```python
from build123d import *

# Parameters (mm, degrees)
PAD001_DEPTH      = 11
FILLET001_R       = 1.2
SKETCH005_W       = 6.70052
SKETCH005_H       = 40.2844
SKETCH006_R       = 5.25
POCKET_DEPTH      = 0.001
POCKET_DEPTH_BACK = 143.4094


with BuildPart() as part:
    # Sketch004 → Pad001 (new body)
    with BuildSketch(Plane.XZ.offset(-6.7)):
        with BuildLine():
            Line((-6.70052, 141.8844), (-9.6647, 143.4084))
            ThreePointArc((-9.6647, 143.4084), (-17.256712, 140.927389), (-24.479189, 137.517128))
            ThreePointArc((-24.479189, 137.517128), (-25.118047, 135.6415), (-23.310129, 134.830602))
            ThreePointArc((-6.70052, 127), (-13.446839, 134.221029), (-23.310129, 134.830602))
            Line((0, 127), (-6.70052, 127))
            Line((0, 141.8844), (0, 127))
            Line((-6.70052, 141.8844), (0, 141.8844))
        make_face()
    pad001 = extrude(amount=PAD001_DEPTH)

    # Mirrored: Pad001 across Sketch004 V_Axis
    add(pad001.mirror(Plane(origin=(0, 6.7, 0), x_dir=(0, -1, 0), z_dir=(1, 0, 0))))

    # Fillet001
    fillet001_edges = [part.edges().sort_by_distance(p)[0] for p in [
        (17.256712, 6.7, 140.927389),
        (17.256712, -4.3, 140.927389),
        (-17.256712, -4.3, 140.927389),
        (-17.256712, 6.7, 140.927389),
    ]]
    fillet(fillet001_edges, radius=FILLET001_R)

    # Sketch005 → Revolution (revolve)
    with BuildSketch(Plane.XZ):
        with Locations((-3.35026, 121.7422)):
            Rectangle(SKETCH005_W, SKETCH005_H)
    revolve(axis=Axis((0, 0, 0), (0, 0, 1)))

    # Sketch006 → Pocket (cut, two sides)
    with BuildSketch(Plane.XY) as pocket_sk:
        Circle(SKETCH006_R)
    extrude(amount=-POCKET_DEPTH, mode=Mode.SUBTRACT)
    extrude(pocket_sk.sketch, amount=POCKET_DEPTH_BACK, mode=Mode.SUBTRACT)


solid = part.part
```
Here's how the part is built. I have some questions about the finished solid (model axes, mm). A direction names the side the tool comes from. Coordinates: 2 decimals unless noted, no trailing zeros. Loops run counter-clockwise (first coordinate to the right, second up) from the corner with the lowest first, then second, coordinate; pieces in that order, holes last. Notation, with made-up numbers: M -39.75,11.25 L -22.75,11.25 A29 ccw -22.75,38.25 Z; hole C -4,45 d8. An arc over 180 degrees is marked long. One line per item, written item: value.
1. Thinking about a two-plate mould opening in X: for faces 1 (the flat face through (7, 6.7, 137)), 2 (the flat face through (-8.162, 1.277, 142.636)), 3 (the cylindrical face through (0.872, -6.644, 117.548)), which applies, +X half, -X half, draft (parallel to the pull), parting line (faces both ways), or undercut?
Geometry says:
face 1: draft
face 2: undercut
face 3: parting line
2. Will these pins go through, and if not, where does the flat tip stop? pin 1 Ø2 at (x, y) = (2, 4) entering from -Z; pin 2 Ø5 at (y, z) = (-1, 107) entering from +X; pin 3 Ø6.5 at (x, y) = (0.5, 2.5) entering from +Z; pin 4 Ø8 at (x, z) = (-14.5, 137.5) entering from -Y.
Geometry says:
pin 1: stops at z = 101.6
pin 2: stops at x = 6.7
pin 3: stops at z = 141.88
pin 4: stops at y = -4.3
3. Imagine slicing it at C-C (y = 4.25). List the corners of the cut face in (x, z) for me.
Geometry says:
outline: M -24.48,137.52 A1.47 ccw -23.31,134.83 A13.36 cw -6.7,127 L -5.18,127 L -5.18,101.6 L -3.08,101.6 L -3.08,141.88 L -6.7,141.88 L -9.66,143.41 A63.79 ccw Z; M 3.08,101.6 L 5.18,101.6 L 5.18,127 L 6.7,127 A13.36 cw 23.31,134.83 A1.47 ccw 24.48,137.52 A63.79 ccw 9.66,143.41 L 6.7,141.88 L 3.08,141.88 Z
4. Imagine slicing it at B-B (z = 125). List the corners of the cut face in (x, y) for me.
Geometry says:
outline: C 0,0 d13.4; hole C 0,0 d10.5
5. On a 3-axis mill with a long thin cutter (end or side, diameter ignored), from which of +Z, -Z, +X, -X, +Y, -Y can I reach the whole of each face in a straight line? I mean faces 4 (the flat face through (-5, 5, 127)), 5 (the flat face through (8.162, 1.277, 142.636)), 6 (the flat face through (-6.2, -3.1, 127)). Say none if no direction works.
Geometry says:
face 4: -Z, -X, +Y
face 5: +Z, +Y, -Y
face 6: -Z, -X, -Y
6. Please list where these lines run through material, in increasing order: probe 1 along X at (y, z) = (0, 113.5); probe 2 along Y at (x, z) = (18, 138).
Geometry says:
probe 1: x = -6.7 to -5.25, 5.25 to 6.7
probe 2: y = -4.3 to 6.7
7. Imagine slicing it at A-A (y = 1). List the corners of the cut face in (x, z) for me.
Geometry says:
outline: M -24.48,137.52 A1.47 ccw -23.31,134.83 A13.36 cw -6.7,127 L -6.63,127 L -6.63,101.6 L -5.15,101.6 L -5.15,141.88 L -6.7,141.88 L -9.66,143.41 A63.79 ccw Z; M 5.15,101.6 L 6.63,101.6 L 6.63,127 L 6.7,127 A13.36 cw 23.31,134.83 A1.47 ccw 24.48,137.52 A63.79 ccw 9.66,143.41 L 6.7,141.88 L 5.15,141.88 Z
